from build123d import *

# Parameters (mm, degrees)
EXTRUDE_1_DEPTH     = 76
SKETCH_2_W          = 66
SKETCH_2_H          = 15
CUT_EXTRUDE_1_DEPTH = 109.200046211


with BuildPart() as part:
    # Эскиз1 → Бобышка-Вытянуть1 (new body)
    with BuildSketch(Plane.XY):
        Polygon((37.5, 2.5), (17.5, 17.5), (-17.5, 17.5), (-17.5, 10.5), (-37.5, 10.5), (-37.5, -7.5), (19.5, -7.5), (19.5, -17.5), (31.5, -17.5), (31.5, -7.5), (37.5, -7.5), align=None)
    extrude(amount=EXTRUDE_1_DEPTH)

    # Эскиз2 → Вырез-Вытянуть1 (cut, through all)
    with BuildSketch(Plane(origin=(37.5, 0, 0), x_dir=(0, 0, -1), z_dir=(1, 0, 0))):
        with Locations((-38, 10)):
            Rectangle(SKETCH_2_W, SKETCH_2_H)
    extrude(amount=-CUT_EXTRUDE_1_DEPTH, mode=Mode.SUBTRACT)


solid = part.part
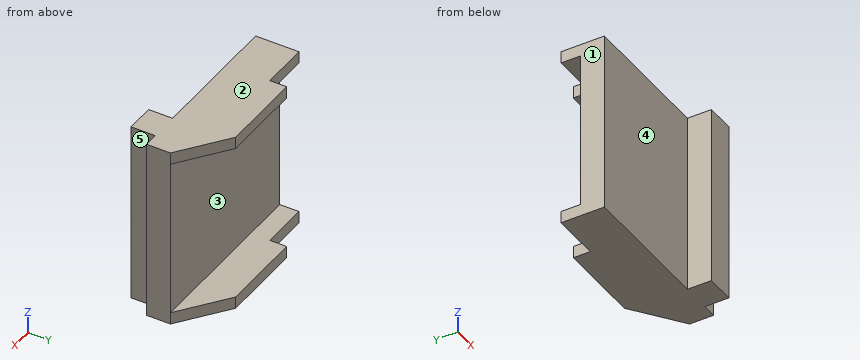
CAD build for the part. Positions are in the model's coordinates, mm. Face numbers are marked on the shaded views. A direction names the side the tool comes from. Coordinates: 2 decimals unless noted, no trailing zeros. Order: outer loops, then holes, each group sorted by start corner. A loop starts at its lowest first (then second) coordinate and runs counter-clockwise, first axis right, second up.
Item 1: Band-saw the part on A-A on y = 5.5. List the corners of the cut face in (x, z).
Check sheet entries:
outline: (-37.5, 0) - (33.5, 0) - (33.5, 5) - (-37.5, 5) - close; (-37.5, 71) - (33.5, 71) - (33.5, 76) - (-37.5, 76) - close
Item 2: Band-saw the part on D-D on y = 12. List the corners of the cut face in (x, z), plus the area to 3 significant figures.
Check sheet entries:
outline: (-17.5, 0) - (24.83, 0) - (24.83, 5) - (-17.5, 5) - close; (-17.5, 71) - (24.83, 71) - (24.83, 76) - (-17.5, 76) - close
area: 423 mm2
Item 3: 3-axis set-ups, long thin cutter, end or side, ignore diameter. For the marked faces 1, 2, 3, 4 and 5: which of +Z, -Z, +X, -X, +Y, -Y reach the whole face in a straight line?
Check sheet entries:
face 1: +Z, -Z, -X, +Y, -Y
face 2: +Z, +X, -X, +Y, -Y
face 3: +X, -X, +Y
face 4: +Z, -Z, -X, -Y
face 5: +Z, -Z, +X, -Y
Item 4: Band-saw the part on B-B on x = -14.5. List the corners of the cut face in (y, z), plus the area to 3 significant figures.
Check sheet entries:
outline: (-7.5, 0) - (17.5, 0) - (17.5, 5) - (2.5, 5) - (2.5, 71) - (17.5, 71) - (17.5, 76) - (-7.5, 76) - close
area: 910 mm2
Item 5: Pin check, flat tips, straight feed: pin 1 Ø5 at (x, z) = (34.5, 54.5) entering from -Y; pin 2 Ø2 at (x, z) = (6, 34) entering from +Y; pin 3 Ø8 at (y, z) = (-13.5, 34.5) entering from -X; pin 4 Ø8 at (x, y) = (-20.5, -12.5) entering from -Z. Stop position of each tip, or through.
Check sheet entries:
pin 1: stops at y = -7.5
pin 2: stops at y = 2.5
pin 3: stops at x = 19.5
pin 4: passes through
Item 6: Band-saw the part on C-C on z = 21.5. List the corners of the cut face in (x, y), plus the area to 3 significant figures.
Check sheet entries:
outline: (-37.5, -7.5) - (19.5, -7.5) - (19.5, -17.5) - (31.5, -17.5) - (31.5, -7.5) - (37.5, -7.5) - (37.5, 2.5) - (-37.5, 2.5) - close
area: 870 mm2
Item 7: Drill centre lines: L1, parallel to Z at x = 21.5, y = 13; L2, parallel to Y at x = -17, z = 8; L3, parallel to X at y = -12, z = 15.5. Where is each one in solid material? Low to high.
Check sheet entries:
L1: z = 0 to 5, 71 to 76
L2: y = -7.5 to 2.5
L3: x = 19.5 to 31.5
